Source: three-view drawing plus pictorial views. Frame: mm from the lowest corner of the part. A direction names the side the tool comes from. Give positions to 0.01 mm unless a question says otherwise; leave off trailing zeros. Loops run counter-clockwise (first coordinate to the right, second up) from the corner with the lowest first, then second, coordinate; pieces in that order, holes last.
1. Material intervals for line 1 along Y through (x, z) = (59, 6.35); line 2 along X through (y, z) = (14, 1.75); line 3 along X through (y, z) = (4, 7), sorted ascending.
2. First-contact query: P1, Ø5, axis at y = 4.5, z = 2, coming from the +X side; P2, Ø3.5, axis at y = 13, z = 2, coming from the -X side; P3, Ø4, axis at x = 55, z = 6, coming from the -Y side; P4, Ø1.5, axis at x = 13.5, y = 12, coming from the -Z side. Flat tips, straight axial feed; report the tip coordinate or a pass-through.
3. Draft query along Y for the marked faces 1, 2, 3 and 4. Return one class per face: +Y half, -Y half, draft (parallel to the pull), parting line (faces both ways), or undercut.
4. Section B-B, the plane y = 10.25. State how many separate pieces and enclosed holes the cut face has, then the cut area to 3 significant figures.
5. Section D-D, the plane x = 7.5. Output: boundary loops of the cut face in (y, z).
6. Section C-C, the plane y = 5.75. Output: boundary loops of the cut face in (x, z), then the cut area to 3 significant figures.
7. Access query for the marked faces 5, 6 and 7. Directions: +Z, -Z, +X, -X, +Y, -Y. A direction counts if a zero-diameter tool reaches every point of the face in a straight line with its end or side. Return the directions, or none.
8. Section A-A, the plane x = 34. Output: boundary loops of the cut face in (y, z), then the cut area to 3 significant figures.
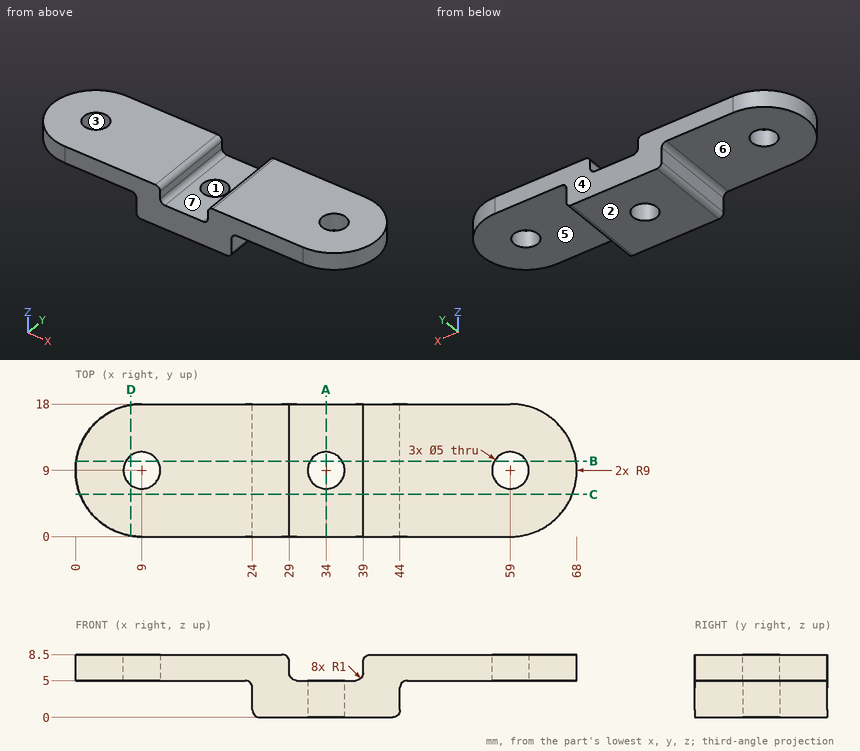
Answers below:
1. line 1: y = 0 to 6.5, 11.5 to 18
1. line 2: x = 24 to 44
1. line 3: x = 1.52 to 29, 39 to 66.48
2. P1: stops at x = 44.13
2. P2: stops at x = 24
2. P3: stops at y = 0
2. P4: stops at z = 5
3. face 1: undercut
3. face 2: draft
3. face 3: undercut
3. face 4: +Y half
4. separate pieces: 4
4. enclosed holes: 0
4. area: 250 mm2
5. outline: (0.13, 5) - (7, 5) - (7, 8.5) - (0.13, 8.5) - close; (11, 5) - (17.87, 5) - (17.87, 8.5) - (11, 8.5) - close
6. outline: (0.61, 5) - (23, 5) arc R1 cw to (24, 4) - (24, 1) arc R1 ccw to (25, 0) - (43, 0) arc R1 ccw to (44, 1) - (44, 4) arc R1 cw to (45, 5) - (67.39, 5) - (67.39, 8.5) - (40, 8.5) arc R1 ccw to (39, 7.5) - (39, 6) arc R1 cw to (38, 5) - (30, 5) arc R1 cw to (29, 6) - (29, 7.5) arc R1 ccw to (28, 8.5) - (0.61, 8.5) - close
6. area: 299 mm2
7. face 5: -Z, +X, +Y, -Y
7. face 6: -Z, -X, +Y, -Y
7. face 7: +Z, +Y, -Y
8. outline: (0, 0) - (6.5, 0) - (6.5, 5) - (0, 5) - close; (11.5, 0) - (18, 0) - (18, 5) - (11.5, 5) - close
8. area: 65.0 mm2
